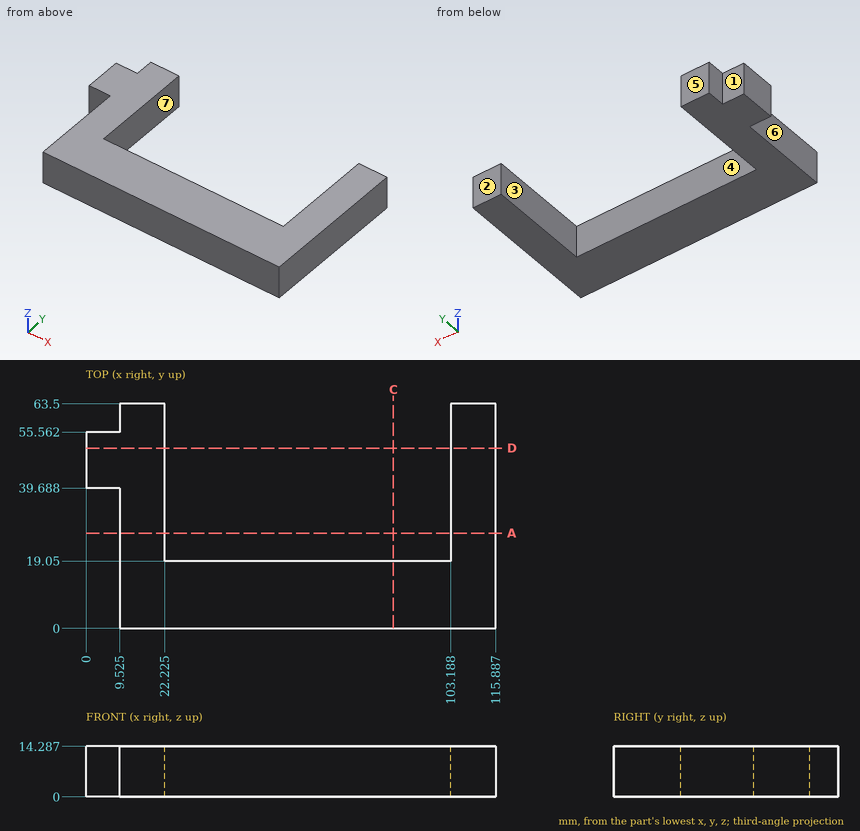
Here's the drawing with two shaded views (mm, measured from the low corner). I have some questions. A direction names the side the tool comes from. Coordinates: 2 decimals unless noted, no trailing zeros. Order: outer loops, then holes, each group sorted by start corner. A loop starts at its lowest first (then second) coordinate and runs counter-clockwise, first axis right, second up. Notation, with made-up numbers: (-13, 45) - (-1, 45) arc R22 ccw to (-1, 67) - close; hole circle Ø7 at (22, -9). An arc over 180 degrees is marked (long way). Answer in a Markdown table with one row per item. Add a question column.
(1) If we section it at C-C, the plane x = 87: Please give me the cut outline in (y, z), then the cut area to 3 significant figures.
(2) On a 3-axis mill with a long thin cutter (end or side, diameter ignored), from which of +Z, -Z, +X, -X, +Y, -Y can I reach the whole of each face in a straight line? I mean the marked faces 1, 2 and 3. Say none if no direction works.
(3) I need wall thicknesses on L1, parallel to X at y = 61, z = 6.5 (1 decimal); L2, parallel to X at y = 40, z = 12 (1 decimal); L3, parallel to Y at x = 79.5, z = 3. Which ranges of each line are inside material? Lowest first, please.
(4) If we section it at D-D, the plane y = 51: Please give me the cut outline in (x, z) (1 decimal), then the cut area to 3 significant figures.
(5) If we mould it in two halves opening along X, with no side actions, what happens to the marked faces 4, 5, 6 and 7? For each: released by +X, released by -X, zero draft, split by the parting line, or undercut.
(6) Will these pins go through, and if not, where does the flat tip stop? pin 1 (7 mm diameter, centred on x = 78, z = 4.5, fed in from +Y); pin 2 (6.5 mm diameter, centred on y = 61, z = 9, fed in from -X) (1 decimal); pin 3 (3 mm diameter, centred on x = 2.5, z = 8, fed in from -Y).
(7) If we section it at A-A, the plane y = 27: Please give me the cut outline in (x, z) (1 decimal), then the cut area to 3 significant figures.
Results are:
| question | item | result |
|---|---|---|
| 1 | outline | (0, 0) - (19.05, 0) - (19.05, 14.29) - (0, 14.29) - close |
| 1 | area | 272 mm2 |
| 2 | face 1 | +Z, -Z, -X, +Y |
| 2 | face 2 | +Z, -Z, +X, -X, +Y |
| 2 | face 3 | +Z, -Z, +Y |
| 3 | L1 | x = 9.5 to 22.2, 103.2 to 115.9 |
| 3 | L2 | x = 0 to 22.2, 103.2 to 115.9 |
| 3 | L3 | y = 0 to 19.05 |
| 4 | outline | (0, 0) - (22.2, 0) - (22.2, 14.3) - (0, 14.3) - close; (103.2, 0) - (115.9, 0) - (115.9, 14.3) - (103.2, 14.3) - close |
| 4 | area | 499 mm2 |
| 5 | face 4 | undercut |
| 5 | face 5 | zero draft |
| 5 | face 6 | released by -X |
| 5 | face 7 | undercut |
| 6 | pin 1 | stops at y = 19.05 |
| 6 | pin 2 | stops at x = 9.5 |
| 6 | pin 3 | stops at y = 39.69 |
| 7 | outline | (9.5, 0) - (22.2, 0) - (22.2, 14.3) - (9.5, 14.3) - close; (103.2, 0) - (115.9, 0) - (115.9, 14.3) - (103.2, 14.3) - close |
| 7 | area | 363 mm2 |
